Part print with two shaded views. Sizes in mm from the minimum x, y, z corner. Round coordinates to 2 decimals unless told otherwise and drop trailing zeros. Loops run counter-clockwise (first coordinate to the right, second up) from the corner with the lowest first, then second, coordinate; pieces in that order, holes last. Notation, with made-up numbers: (19, 23.25) - (35, 23.25) arc R26 cw to (35, 41.25) - close; hole circle Ø2 at (-19.5, -9.5). An arc over 180 degrees is marked (long way). One line per question, with ' | ' between items.
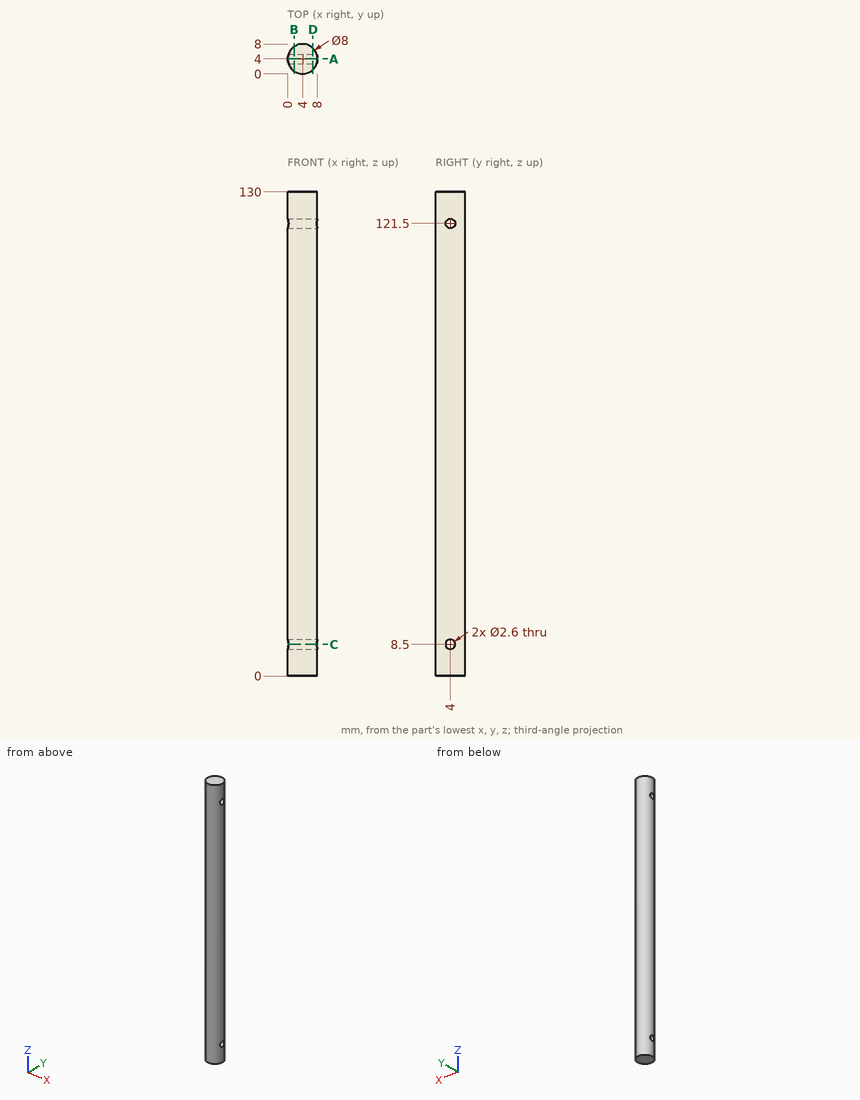
(1) Cut at D-D, the plane x = 6.75. Write the cut outline in (y, z).
Results found:
outline: (1.1, 0) - (6.9, 0) - (6.9, 130) - (1.1, 130) - close; hole circle Ø2.6 at (4, 8.5); hole circle Ø2.6 at (4, 121.5)
(2) Cut at A-A, the plane y = 4. Write the cut outline in (x, z).
Results found:
outline: (0, 0) - (8, 0) - (8, 7.2) - (0, 7.2) - close; (0, 9.8) - (8, 9.8) - (8, 120.2) - (0, 120.2) - close; (0, 122.8) - (8, 122.8) - (8, 130) - (0, 130) - close
(3) Cut at C-C, the plane z = 8.5. Write the cut outline in (x, y).
Results found:
outline: (0.22, 2.7) arc R4 ccw to (7.78, 2.7) - close; (0.22, 5.3) - (7.78, 5.3) arc R4 ccw to start
(4) Probe L1, parallel to Z at x = 6, y = 4.25; L2, parallel to Z at x = 5.5, y = 3.5; L3, parallel to Y at x = 3.75, z = 121.5. List the from-to ranges inside material, lowest first.
Results found:
L1: z = 0 to 7.22, 9.78 to 120.22, 122.78 to 130 | L2: z = 0 to 7.3, 9.7 to 120.3, 122.7 to 130 | L3: y = 0.01 to 2.7, 5.3 to 7.99
(5) Cut at B-B, the plane x = 1.75. Write the cut outline in (y, z).
Results found:
outline: (0.69, 0) - (7.31, 0) - (7.31, 130) - (0.69, 130) - close; hole circle Ø2.6 at (4, 8.5); hole circle Ø2.6 at (4, 121.5)
